Source: CAD feature listing. Evaluate the final solid. Frame: model axes, mm. A direction names the side the tool comes from. Coordinates: 2 decimals unless noted, no trailing zeros. Order: outer loops, then holes, each group sorted by start corner. A loop starts at its lowest first (then second) coordinate and runs counter-clockwise, first axis right, second up.
Item 1: Section D-D on y = 5.5. Return the cut outline in (x, z), then the cut area to 3 significant figures.
Item 2: Section B-B on z = 0. Return the cut outline in (x, y).
Item 3: Mould query, pull axis X, two halves, no side actions, for faces 3 (the cylindrical face through (-29.97, 3.45, -1.32)), 4 (the flat face through (6, 7, 0)), 5 (the flat face through (24.26, 5.52, 14.04)). Classes: released by +X, released by -X, zero draft, split by the parting line, or undercut.
Item 4: Section A-A on x = 0. Return the cut outline in (y, z).
Item 5: Ray query, line 1 (Z direction, x = 0, y = 1.8); line 2 (X direction, y = 4.75, z = 12); line 3 (Z direction, x = 0, y = 4.7). Return the intervals inside material, ascending.
Item 6: Section C-C on y = 2. Return the cut outline in (x, z).
Item 7: Reachability of faces 1 (the flat face through (-19.04, 5.52, 14.04)), 2 (the cylindrical face through (-23.45, 1.97, 12.42)) from +Z, -Z, +X, -X, +Y, -Y: full face, straight path, thin tool, end or side. Return the list, or none.
Item 8: Contact query for flat-ended pins moving along their axis: P1, Ø2.5, axis at x = 22.5, y = 5, coming from the +Z side; P2, Ø2.5, axis at x = -21.5, y = 5.5, coming from the -Z side; P3, Ø3.5, axis at x = -21, y = 5.5, coming from the +Z side; P4, Ø5, axis at x = 0.5, z = -23.5, coming from the +Y side. Output: stop coordinate, or through.
from build123d import *

# Parameters (mm, degrees)
SKETCH1_R           = 30
SKETCH1_R_2         = 1.8
BOSS_EXTRUDE1_DEPTH = 7
SKETCH2_R           = 3.75
CUT_EXTRUDE1_DEPTH  = 3


with BuildPart() as part:
    # Sketch1 → Boss-Extrude1 (new body)
    with BuildSketch(Plane(origin=(0, 0, 0), x_dir=(1, 0, 0), z_dir=(0, 1, 0))):
        Circle(SKETCH1_R)
        Circle(SKETCH1_R_2, mode=Mode.SUBTRACT)
        with Locations((0, 25)):
            Circle(SKETCH1_R_2, mode=Mode.SUBTRACT)
        with Locations((21.650635095, -12.5)):
            Circle(SKETCH1_R_2, mode=Mode.SUBTRACT)
        with Locations((-21.650635095, -12.5)):
            Circle(SKETCH1_R_2, mode=Mode.SUBTRACT)
    extrude(amount=BOSS_EXTRUDE1_DEPTH)

    # Sketch2 → Cut-Extrude1 (cut)
    with BuildSketch(Plane(origin=(0, 7, 0), x_dir=(1, 0, 0), z_dir=(0, 1, 0))):
        Circle(SKETCH2_R)
        Polygon((19.900635095, -15.531088913), (23.400635095, -15.531088913), (25.150635095, -12.5), (23.400635095, -9.468911087), (19.900635095, -9.468911087), (18.150635095, -12.5), align=None)
        Polygon((3.5, 25), (1.75, 28.031088913), (-1.75, 28.031088913), (-3.5, 25), (-1.75, 21.968911087), (1.75, 21.968911087), align=None)
        Polygon((-23.400635095, -9.468911087), (-25.150635095, -12.5), (-23.400635095, -15.531088913), (-19.900635095, -15.531088913), (-18.150635095, -12.5), (-19.900635095, -9.468911087), align=None)
    extrude(amount=-CUT_EXTRUDE1_DEPTH, mode=Mode.SUBTRACT)


solid = part.part
Answer list:
1. outline: circle Ø60 at (0, 0); hole (-25.15, 12.5) - (-23.4, 9.47) - (-19.9, 9.47) - (-18.15, 12.5) - (-19.9, 15.53) - (-23.4, 15.53) - close; hole circle Ø7.5 at (0, 0); hole (-3.5, -25) - (-1.75, -28.03) - (1.75, -28.03) - (3.5, -25) - (1.75, -21.97) - (-1.75, -21.97) - close; hole (18.15, 12.5) - (19.9, 9.47) - (23.4, 9.47) - (25.15, 12.5) - (23.4, 15.53) - (19.9, 15.53) - close
1. area: 2,690 mm2
2. outline: (-30, 0) - (-1.8, 0) - (-1.8, 4) - (-3.75, 4) - (-3.75, 7) - (-30, 7) - close; (1.8, 0) - (30, 0) - (30, 7) - (3.75, 7) - (3.75, 4) - (1.8, 4) - close
3. face 3: split by the parting line
3. face 4: zero draft
3. face 5: undercut
4. outline: (0, -30) - (7, -30) - (7, -28.03) - (4, -28.03) - (4, -26.8) - (0, -26.8) - close; (0, -23.2) - (4, -23.2) - (4, -21.97) - (7, -21.97) - (7, -3.75) - (4, -3.75) - (4, -1.8) - (0, -1.8) - close; (0, 1.8) - (4, 1.8) - (4, 3.75) - (7, 3.75) - (7, 30) - (0, 30) - close
5. line 1: z = -30 to -26.8, -23.2 to -1.8, 1.8 to 30
5. line 2: x = -27.5 to -24.86, -18.44 to 18.44, 24.86 to 27.5
5. line 3: z = -30 to -28.03, -21.97 to -3.75, 3.75 to 30
6. outline: circle Ø60 at (0, 0); hole circle Ø3.6 at (-21.65, 12.5); hole circle Ø3.6 at (0, -25); hole circle Ø3.6 at (0, 0); hole circle Ø3.6 at (21.65, 12.5)
7. face 1: +Y
7. face 2: +Y, -Y
8. P1: stops at z = 21.18
8. P2: stops at z = -22.13
8. P3: stops at z = 23.01
8. P4: stops at y = 7
